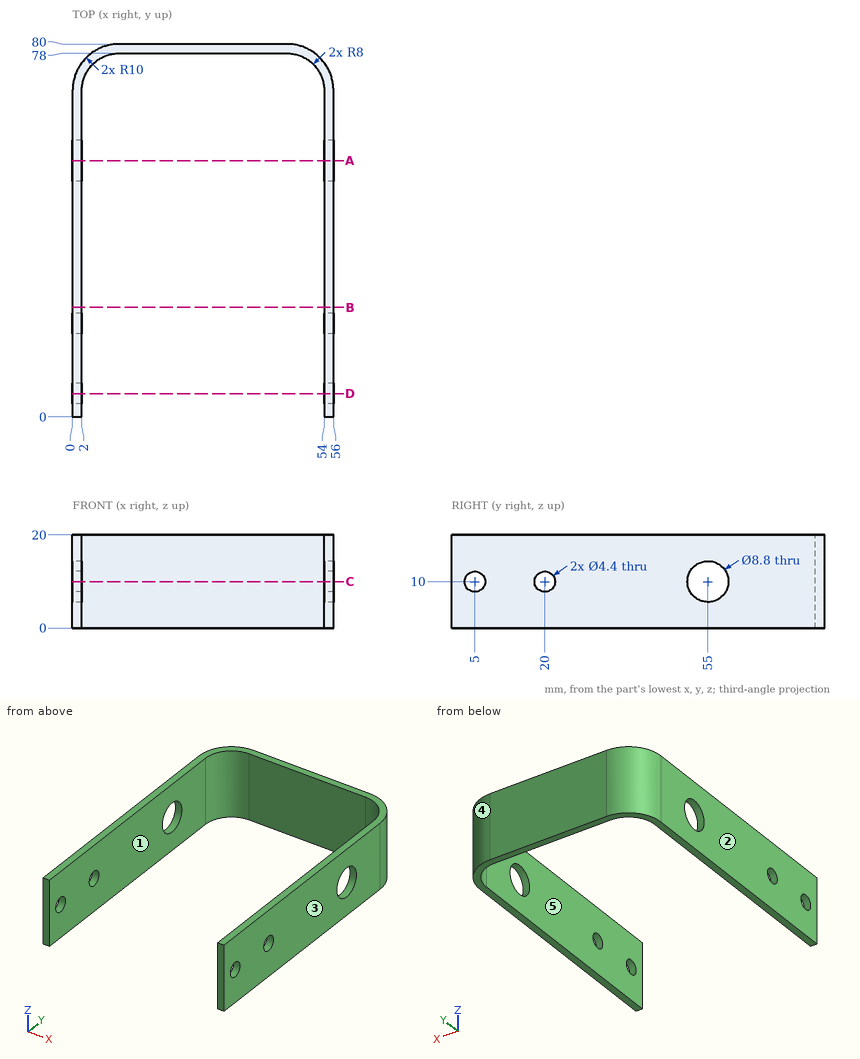
Study the drawing (mm; zero at the part's minimum x, y, z) and answer. A direction names the side the tool comes from. Coordinates: 2 decimals unless noted, no trailing zeros. Write each loop counter-clockwise with the first axis right and the second up, starting at its lowest first coordinate (ties: lowest second). Pieces come first, ordered by that corner, then holes. Notation, with made-up numbers: (83.5, 17.5) - (112.5, 17.5) arc R19 ccw to (112.5, 34.5) - close; hole circle Ø1 at (56.5, 76.25). An arc over 180 degrees is marked (long way). One line per item, written item: value.
1) Find section A-A (y = 55). Give the vertices of the cut face in (x, z), and give its area (3 significant figures).
Geometry check:
outline: (0, 0) - (2, 0) - (2, 5.6) - (0, 5.6) - close; (0, 14.4) - (2, 14.4) - (2, 20) - (0, 20) - close; (54, 0) - (56, 0) - (56, 5.6) - (54, 5.6) - close; (54, 14.4) - (56, 14.4) - (56, 20) - (54, 20) - close
area: 44.8 mm2
2) A tool of negligible diameter and unlimited length cuts with its end or side. For the marked faces 4 and 5, from which of +Z, -Z, +X, -X, +Y, -Y can it reach the whole face along a straight path? Write none if from no direction.
Geometry check:
face 4: +Z, -Z, +X, +Y
face 5: +Z, -Z, -Y
3) Find section C-C (z = 10). Count the separate pieces of the cut face and the enclosed holes in it, and give its area (3 significant figures).
Geometry check:
separate pieces: 7
enclosed holes: 0
area: 338 mm2
4) This flat-tipped pin is pushed along its axis until it touches: pin 1 Ø3 at (x, z) = (45, 10.5) entering from -Y. Where does it stop, or does it pass through?
Geometry check:
pin 1: stops at y = 77.98
5) Consider line 1 along X through (y, z) = (63, 3.5); line 2 along Z through (x, y) = (1, 55); line 3 along Z through (x, y) = (0.75, 20). Determine where each line is inside the solid, lowest interval first. Write a range as from..to.
Geometry check:
line 1: x = 0..2, 54..56
line 2: z = 0..5.6, 14.4..20
line 3: z = 0..7.8, 12.2..20
6) For a pull along X with two mould halves and no side action, classify the marked faces 1, 2 and 3 as pulls with the +X half, pulls with the -X half, needs draft (parallel to the pull), parting line crosses it, or undercut.
Geometry check:
face 1: undercut
face 2: pulls with the -X half
face 3: pulls with the +X half
7) Find section B-B (y = 23.5). Give the vertices of the cut face in (x, z).
Geometry check:
outline: (0, 0) - (2, 0) - (2, 20) - (0, 20) - close; (54, 0) - (56, 0) - (56, 20) - (54, 20) - close
8) Find section D-D (y = 5). Give the vertices of the cut face in (x, z), and give its area (3 significant figures).
Geometry check:
outline: (0, 0) - (2, 0) - (2, 7.8) - (0, 7.8) - close; (0, 12.2) - (2, 12.2) - (2, 20) - (0, 20) - close; (54, 0) - (56, 0) - (56, 7.8) - (54, 7.8) - close; (54, 12.2) - (56, 12.2) - (56, 20) - (54, 20) - close
area: 62.4 mm2
